The listing builds one solid part. Answer for the finished solid, in the listing's coordinates (mm). A direction names the side the tool comes from. Coordinates: 2 decimals unless noted, no trailing zeros. Order: outer loops, then holes, each group sorted by start corner. A loop starts at its lowest first (then second) coordinate and runs counter-clockwise, first axis right, second up. Notation, with made-up numbers: (15.25, 2.25) -> (26.25, 2.25) arc R30 ccw to (26.25, 38.25) -> close; hole circle Ø10 at (50, 53.25). An arc over 180 degrees is marked (long way). Return JSON: item names as keys, results as strings.
Autodesk Inventor part; units mm, degrees
ref_plane "YZ Plane" through (0, 0, 0) normal (1, 0, 0) x (0, 1, 0)
ref_plane "XZ Plane" through (0, 0, 0) normal (0, 1, 0) x (-1, 0, 0)
ref_plane "XY Plane" through (0, 0, 0) normal (0, 0, 1) x (1, 0, 0)
sketch "Skizze1" plane through (0, 0, 0) normal (0, 0, 1) x (1, 0, 0)
  line L0 (0, 0) -> (53, 0)
  line L1 (53, 0) -> (53, 30)
  line L2 (53, 30) -> (0, 30)
  line L3 (0, 30) -> (0, 0)
  dimension "d0" = 30
  dimension "d1" = 53
extrude "Extrusion1" add sketch "Skizze1" along normal blind 2
sketch "Skizze2" plane through (0, 0, 2) normal (0, 0, 1) x (1, 0, 0)
  line L0 (0, 0) -> (53, 0)
  line L1 (53, 0) -> (53, 30)
  line L2 (53, 30) -> (0, 30)
  line L3 (0, 30) -> (0, 0)
  line L4 (2.5, 2.5) -> (50.5, 2.5)
  line L5 (50.5, 2.5) -> (50.5, 27.5)
  line L6 (50.5, 27.5) -> (2.5, 27.5)
  line L7 (2.5, 27.5) -> (2.5, 2.5)
  dimension "d4" = 25
  dimension "d5" = 48
  dimension "d6" = 2.5
  dimension "d7" = 2.5
  dimension "d8" = 2.5
  dimension "d9" = 2.5
extrude "Extrusion2" add sketch "Skizze2" along normal blind 12
sketch "Skizze3" plane through (0, 0, 2) normal (0, 0, 1) x (1, 0, 0)
  line L0 (10, 18.5) -> (40, 18.5)
  line L1 (40, 18.5) -> (40, 11.5)
  line L2 (40, 11.5) -> (10, 11.5)
  line L3 (10, 11.5) -> (10, 18.5)
  line L4 (0, 30) -> (0, 0)
  line L5 (50.5, 27.5) -> (2.5, 27.5)
  line L6 (2.5, 2.5) -> (50.5, 2.5)
  dimension "d12" = 10
  dimension "d13" = 30
  dimension "d14" = 7
  dimension "d15" = 9
  dimension "d16" = 9
extrude "Extrusion3" add sketch "Skizze3" along normal blind 7
hole "Bohrung1" at (17.5, 15, 9) direction (0, 0, -1) diameter 3.2 end through all
sketch "Skizze4" plane through (0, 0, 0) normal (0, 0, -1) x (-1, 0, 0)
  line L0 (-19.3149, 18.0854) -> (-15.7355, 18.1144)
  line L1 (-15.7355, 18.1144) -> (-13.9205, 15.0291)
  line L2 (-13.9205, 15.0291) -> (-15.6851, 11.9146)
  line L3 (-15.6851, 11.9146) -> (-19.2645, 11.8856)
  line L4 (-19.2645, 11.8856) -> (-21.0795, 14.9709)
  line L5 (-21.0795, 14.9709) -> (-19.3149, 18.0854)
  line L6 (-2.5, 2.5) -> (-50.5, 2.5)
  line L7 (-2.5, 27.5) -> (-2.5, 2.5)
  point P0 (0, 0)
  point P1 (-17.5, 15)
  dimension "d28" = 6.2
  dimension "d29" = 12.5
  dimension "d30" = 15
extrude "Extrusion4" cut sketch "Skizze4" against normal blind 5
sketch "Skizze5" plane through (0, 0, 9) normal (0, 0, 1) x (1, 0, 0)
  circle A0 centre (17.5, 15) radius 2.5
  line L0 (2.5, 2.5) -> (2.5, 27.5)
  line L1 (40, 18.5) -> (10, 18.5)
  circle A1 centre (17.5, 15) radius 1.6
  point P0 (0, 0)
  dimension "d33" = 5
  dimension "d34" = 15
  dimension "d35" = 3.5
extrude "Extrusion5" add sketch "Skizze5" along normal blind 2
sketch "Skizze6" plane through (0, 0, 14) normal (0, 0, 1) x (1, 0, 0)
  line L0 (50.5, 27.5) -> (50.5, 2.5)
  line L1 (53, 0) -> (53, 30)
  line L2 (50.5, 9) -> (53, 9)
  line L3 (53, 9) -> (53, 21)
  line L4 (53, 21) -> (50.5, 21)
  line L5 (50.5, 21) -> (50.5, 9)
  line L6 (0, 0) -> (53, 0)
  line L7 (53, 30) -> (0, 30)
  dimension "d38" = 12
  dimension "d39" = 9
  dimension "d40" = 9
extrude "Extrusion6" add sketch "Skizze6" along normal blind 4
sketch "Skizze7" plane through (0, 0, 14) normal (0, 0, 1) x (1, 0, 0)
  line L0 (0, 30) -> (0, 0)
  line L1 (2.5, 2.5) -> (2.5, 27.5)
  line L2 (0, 12) -> (2.5, 12)
  line L3 (2.5, 12) -> (2.5, 18)
  line L4 (2.5, 18) -> (0, 18)
  line L5 (0, 18) -> (0, 12)
  line L6 (0, 0) -> (53, 0)
  line L7 (53, 30) -> (0, 30)
  dimension "d43" = 6
  dimension "d44" = 12
  dimension "d45" = 12
extrude "Extrusion7" cut sketch "Skizze7" against normal blind 4
fillet "Rundung1" radius 1 4 edges at (51.75, 21, 18) (51.75, 9, 18) (1.25, 18, 10) (1.25, 12, 10)
properties part number "V2_unterteil"
1. For faces 1 (the face through (25, 18.5, 5)), 2 (the face through (52, 21, 15)), 3 (the face through (52, 9, 15)), 4 (the face through (20.16, 13.41, 2.46)), determine the directions among +Z, -Z, +X, -X, +Y, -Y from which every point of the face is accessible in a straight line to the end or side of a thin tool.
Answer block:
{"face 1": "+Z", "face 2": "+Z, +X, -X, +Y", "face 3": "+Z, +X, -X, -Y", "face 4": "-Z"}
2. The part is cut by section C-C on x = 17.5. Give the vertices of the cut face in (y, z), and give its area (3 significant figures).
Answer block:
{"outline": "(0, 0) -> (11.9, 0) -> (11.9, 5) -> (13.4, 5) -> (13.4, 11) -> (12.5, 11) -> (12.5, 9) -> (11.5, 9) -> (11.5, 2) -> (2.5, 2) -> (2.5, 14) -> (0, 14) -> close; (16.6, 5) -> (18.1, 5) -> (18.1, 0) -> (30, 0) -> (30, 14) -> (27.5, 14) -> (27.5, 2) -> (18.5, 2) -> (18.5, 9) -> (17.5, 9) -> (17.5, 11) -> (16.6, 11) -> close", "area": "129 mm2"}
3. The part is cut by section A-A on x = 37.5. Give the vertices of the cut face in (y, z).
Answer block:
{"outline": "(0, 0) -> (30, 0) -> (30, 14) -> (27.5, 14) -> (27.5, 2) -> (18.5, 2) -> (18.5, 9) -> (11.5, 9) -> (11.5, 2) -> (2.5, 2) -> (2.5, 14) -> (0, 14) -> close"}
4. The part is cut by section B-B on y = 25.75. Give the vertices of the cut face in (x, z).
Answer block:
{"outline": "(0, 0) -> (53, 0) -> (53, 14) -> (50.5, 14) -> (50.5, 2) -> (2.5, 2) -> (2.5, 14) -> (0, 14) -> close"}
5. Consider line 1 (Y direction, x = 17.5, z = 7.8); line 2 (X direction, y = 15, z = 6.9); line 3 (X direction, y = 11, z = 6.5). Determine where each line is inside the solid, lowest interval first. Write a range as from..to.
Answer block:
{"line 1": "y = 0..2.5, 11.5..13.4, 16.6..18.5, 27.5..30", "line 2": "x = 0..2.5, 10..15.9, 19.1..40, 50.5..53", "line 3": "x = 0..2.5, 50.5..53"}
6. Determine the mould class of faces 5 (the face through (0, 15, 7)), 6 (the face through (16, 16, 5)), 7 (the face through (52, 15, 18)) for opening direction X: pulls with the +X half, pulls with the -X half, needs draft (parallel to the pull), parting line crosses it, or undercut.
Answer block:
{"face 5": "pulls with the -X half", "face 6": "undercut", "face 7": "needs draft"}
7. Each of these flat-tipped pins is pushed along its axis until it touches: pin 1 Ø4 at (x, y) = (38.5, 18.5) entering from +Z; pin 2 Ø1.5 at (x, y) = (18.5, 16) entering from +Z; pin 3 Ø5.5 at (y, z) = (14.5, 6.5) entering from -X; pin 4 Ø6 at (x, y) = (26, 8) entering from +Z. Where does it stop, or does it pass through?
Answer block:
{"pin 1": "stops at z = 9", "pin 2": "stops at z = 11", "pin 3": "stops at x = 0", "pin 4": "stops at z = 2"}
8. The part is cut by section D-D on y = 15.75. Give the vertices of the cut face in (x, z), and give its area (3 significant figures).
Answer block:
{"outline": "(0, 0) -> (14.34, 0) -> (14.34, 5) -> (16.09, 5) -> (16.09, 11) -> (15.12, 11) -> (15.12, 9) -> (10, 9) -> (10, 2) -> (2.5, 2) -> (2.5, 10) -> (0, 10) -> close; (18.91, 5) -> (20.64, 5) -> (20.64, 0) -> (53, 0) -> (53, 18) -> (50.5, 18) -> (50.5, 2) -> (40, 2) -> (40, 9) -> (19.88, 9) -> (19.88, 11) -> (18.91, 11) -> close", "area": "337 mm2"}
